```python
from build123d import *

# Parameters (mm, degrees)
F0_W     = 160
F0_H     = 200
F1_DEPTH = 3
F2_D     = 5
F4_DEPTH = 25


with BuildPart() as f1:
    # F0 (on Front) → F1 (new body)
    with BuildSketch(Plane.XZ):
        with Locations((0, 100)):
            Rectangle(F0_W, F0_H)
    extrude(amount=F1_DEPTH)

    # F2 (through all)
    with Locations(Plane(origin=(0, 0, 0), x_dir=(1, 0, 0), z_dir=(0, 1, 0))):
        with Locations((47.5, -170), (-47.5, -170), (47.5, -60)):
            Hole(F2_D / 2)

    # F3 (on face) → F4 (cut)
    with BuildSketch(Plane.XZ.offset(3)):
        Polygon((-31.8933982822, 175), (-42.5, 164.3933982822), (-42.5, 0), (42.5, 0), (42.5, 164.3933982822), (31.8933982822, 175), align=None)
    extrude(amount=-F4_DEPTH, mode=Mode.SUBTRACT)


solid = f1.part
```
CAD build for the part. Positions are in the model's coordinates, mm. A direction names the side the tool comes from. Give positions to 0.01 mm unless a question says otherwise; leave off trailing zeros. Write each loop counter-clockwise with the first axis right and the second up, starting at its lowest first coordinate (ties: lowest second). Pieces come first, ordered by that corner, then holes. Notation, with made-up numbers: M 24.25,29 L 66.25,29 A19 ccw 66.25,44 Z; hole C 13,42 d9. An arc over 180 degrees is marked long. Return JSON: item names as keys, results as strings. Group by question number.
(1) Band-saw the part on C-C (y = -0.95). Give the cut face in (x, z), and give its area (3 significant figures).
(2) Flat gauge pins, fed straight in: pin 1 Ø3 at (x, z) = (-47.5, 170) entering from +Y; pin 2 Ø1.5 at (x, y) = (8.5, -2) entering from -Z. Where does each tip first touch, or does it go through?
(3) Band-saw the part on A-A (x = -47.5). Give the cut face in (y, z).
(4) Band-saw the part on B-B (z = 71). Give the cut face in (x, y), and give its area (3 significant figures).
(5) Mould opens along Z. For faces 3 (the face through (-54, 0, 101)), 4 (the face through (47.83, -1.52, 167.52)), 5 (the face through (-37.122, -1.521, 169.771)) say: pulls with the +Z half, pulls with the -Z half, needs draft (parallel to the pull), parting line crosses it, or undercut.
(6) Band-saw the part on D-D (z = 170). Give the cut face in (x, y), and give its area (3 significant figures).
(7) 3-axis set-ups, long thin cutter, end or side, ignore diameter. For faces 1 (the face through (-47.17, -1.52, 167.52)), 2 (the face through (37.271, -1.521, 169.622)): which of +Z, -Z, +X, -X, +Y, -Y reach the whole face in a straight line?
(8) Drill centre lines: L1, parallel to Z at x = 47.5, y = -1.2; L2, parallel to X at y = -2.25, z = 60; L3, parallel to Z at x = -47.5, y = -0.65. Where is each one in solid material? Low to high. Write a range as [from, to].
Entries:
{
 "1": {"outline": "M -80,0 L -42.5,0 L -42.5,164.39 L -31.89,175 L 31.89,175 L 42.5,164.39 L 42.5,0 L 80,0 L 80,200 L -80,200 Z; hole C -47.5,170 d5; hole C 47.5,60 d5; hole C 47.5,170 d5", "area": "17,200 mm^2"},
 "2": {"pin 1": "passes through", "pin 2": "stops at z = 175"},
 "3": {"outline": "M -3,0 L 0,0 L 0,167.5 L -3,167.5 Z; M -3,172.5 L 0,172.5 L 0,200 L -3,200 Z"},
 "4": {"outline": "M -80,-3 L -42.5,-3 L -42.5,0 L -80,0 Z; M 42.5,-3 L 80,-3 L 80,0 L 42.5,0 Z", "area": "225 mm^2"},
 "5": {"face 3": "needs draft", "face 4": "undercut", "face 5": "pulls with the -Z half"},
 "6": {"outline": "M -80,-3 L -50,-3 L -50,0 L -80,0 Z; M -45,-3 L -36.89,-3 L -36.89,0 L -45,0 Z; M 36.89,-3 L 45,-3 L 45,0 L 36.89,0 Z; M 50,-3 L 80,-3 L 80,0 L 50,0 Z", "area": "229 mm^2"},
 "7": {"face 1": "+Y, -Y", "face 2": "-Z, +Y, -Y"},
 "8": {"L1": "z = [0, 57.5], [62.5, 167.5], [172.5, 200]", "L2": "x = [-80, -42.5], [42.5, 45], [50, 80]", "L3": "z = [0, 167.5], [172.5, 200]"}
}
